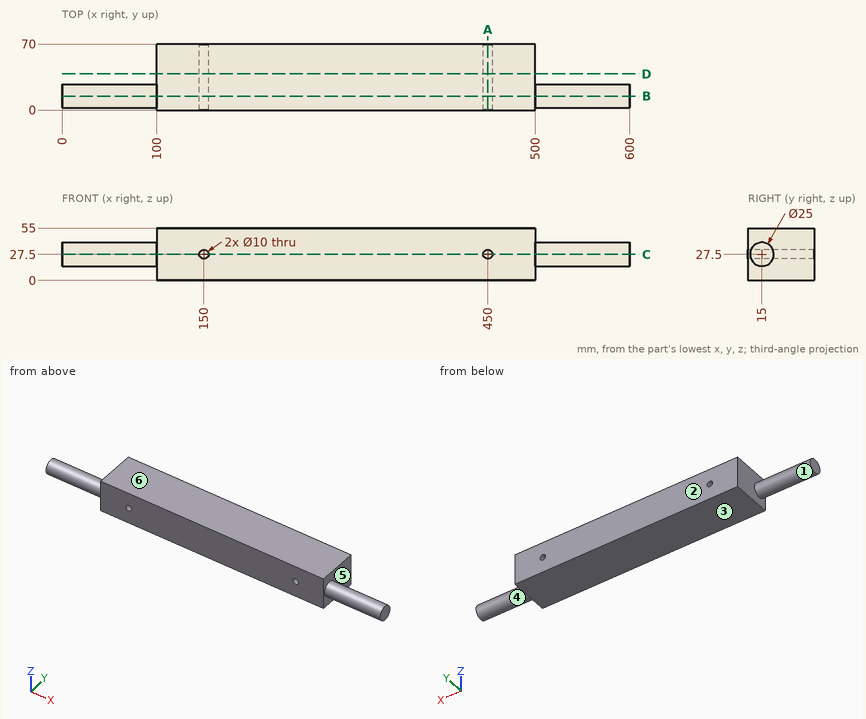
Check sheet for the drawn part. Datum: minimum x, y, z corner. Units: mm. A direction names the side the tool comes from. Coordinates: 2 decimals unless noted, no trailing zeros. Order: outer loops, then holes, each group sorted by start corner. A loop starts at its lowest first (then second) coordinate and runs counter-clockwise, first axis right, second up. Notation, with made-up numbers: (-27, -34) -> (-10, -34) arc R10 cw to (-10, -21) -> close; hole circle Ø1 at (58.5, -4.5). An arc over 180 degrees is marked (long way). Use a Markdown table: item, result. Add a question column.
1. Go/stop test with flat-tipped pins: pin 1 Ø5 at (y, z) = (36, 12.5) entering from -X; pin 2 Ø8 at (x, z) = (450, 27.5) entering from -Y; pin 3 Ø6 at (y, z) = (59.5, 24) entering from +X. Record where each tip stops, or that it passes through.
2. Cross-section at C-C (z = 27.5). Enter the section's corners in (x, y).
3. Material ranges on L1, parallel to X at y = 41.5, z = 27.5; L2, parallel to Z at x = 150, y = 53; L3, parallel to X at y = 30, z = 31.5, recorded low to high.
4. Mould release check, pull along Z, two halves, no side actions. Record for the marked faces 3, 4, 5 and 6: pulls with the +Z half, pulls with the -Z half, needs draft (parallel to the pull), parting line crosses it, or undercut.
5. Set-up check for the marked faces 1 and 2: record each of +Z, -Z, +X, -X, +Y, -Y from which the full face is reachable in a straight line by a thin tool's end or side.
6. Cross-section at A-A (x = 450). Enter the section's corners in (y, z).
7. Cross-section at D-D (y = 38.5). Enter the section's corners in (x, z), and give its area (3 significant figures).
8. Cross-section at B-B (y = 15). Enter the section's corners in (x, z).
Filled sheet:
| question | item | result |
|---|---|---|
| 1 | pin 1 | x = 100 |
| 1 | pin 2 | through |
| 1 | pin 3 | x = 500 |
| 2 | outline | (0, 2.5) -> (100, 2.5) -> (100, 0) -> (145, 0) -> (145, 70) -> (100, 70) -> (100, 27.5) -> (0, 27.5) -> close; (155, 0) -> (445, 0) -> (445, 70) -> (155, 70) -> close; (455, 0) -> (500, 0) -> (500, 2.5) -> (600, 2.5) -> (600, 27.5) -> (500, 27.5) -> (500, 70) -> (455, 70) -> close |
| 3 | L1 | 100 to 145, 155 to 445, 455 to 500 |
| 3 | L2 | 0 to 22.5, 32.5 to 55 |
| 3 | L3 | 100 to 147, 153 to 447, 453 to 500 |
| 4 | face 3 | pulls with the -Z half |
| 4 | face 4 | parting line crosses it |
| 4 | face 5 | needs draft |
| 4 | face 6 | pulls with the +Z half |
| 5 | face 1 | -X |
| 5 | face 2 | +Z, -Z, +X, -X, +Y |
| 6 | outline | (0, 0) -> (70, 0) -> (70, 22.5) -> (0, 22.5) -> close; (0, 32.5) -> (70, 32.5) -> (70, 55) -> (0, 55) -> close |
| 7 | outline | (100, 0) -> (500, 0) -> (500, 55) -> (100, 55) -> close; hole circle Ø10 at (150, 27.5); hole circle Ø10 at (450, 27.5) |
| 7 | area | 21,800 mm2 |
| 8 | outline | (0, 15) -> (100, 15) -> (100, 0) -> (500, 0) -> (500, 15) -> (600, 15) -> (600, 40) -> (500, 40) -> (500, 55) -> (100, 55) -> (100, 40) -> (0, 40) -> close; hole circle Ø10 at (150, 27.5); hole circle Ø10 at (450, 27.5) |
